```python
from build123d import *

# Parameters (mm, degrees)
SKETCH1_W           = 25.4
SKETCH1_H           = 25.4
BOSS_EXTRUDE1_DEPTH = 107.95
SKETCH2_W           = 22.098
SKETCH2_H           = 22.098
CUT_EXTRUDE1_DEPTH  = 114.769602707
SKETCH3_R           = 3.175
CUT_EXTRUDE2_DEPTH  = 114.769602707


with BuildPart() as part:
    # Sketch1 → Boss-Extrude1 (new body)
    with BuildSketch(Plane(origin=(0, 0, 0), x_dir=(1, 0, 0), z_dir=(0, 1, 0))):
        with Locations((12.7, -12.7)):
            Rectangle(SKETCH1_W, SKETCH1_H)
    extrude(amount=BOSS_EXTRUDE1_DEPTH)

    # Sketch2 → Cut-Extrude1 (cut, through all)
    with BuildSketch(Plane(origin=(0, 107.95, 0), x_dir=(1, 0, 0), z_dir=(0, 1, 0))):
        with Locations((12.7, -12.7)):
            Rectangle(SKETCH2_W, SKETCH2_H)
    extrude(amount=-CUT_EXTRUDE1_DEPTH, mode=Mode.SUBTRACT)

    # Sketch3 → Cut-Extrude2 (cut, through all)
    with BuildSketch(Plane.ZY):
        with Locations((12.7, 12.7)):
            Circle(SKETCH3_R)
    extrude(amount=-CUT_EXTRUDE2_DEPTH, mode=Mode.SUBTRACT)


solid = part.part
```
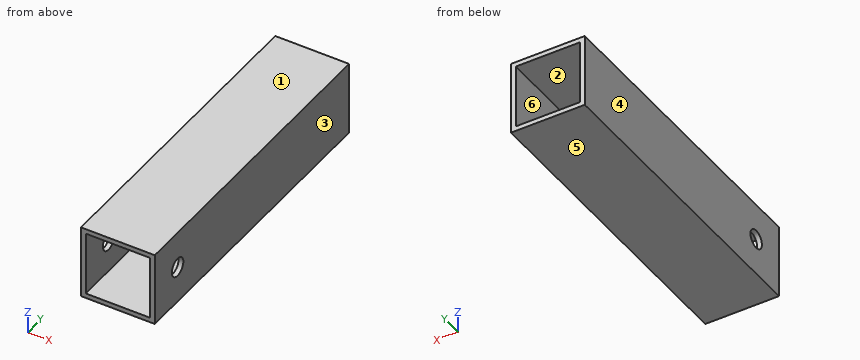
The listing builds one solid part. Answer for the finished solid, in the listing's coordinates (mm). Face numbers are marked on the shaded views. A direction names the side the tool comes from. Coordinates: 2 decimals unless noted, no trailing zeros. Write each loop counter-clockwise with the first axis right and the second up, starting at its lowest first coordinate (ties: lowest second). Pieces come first, ordered by that corner, then holes. Notation, with made-up numbers: (7.5, 81.5) - (62.5, 81.5) arc R8 ccw to (62.5, 92.5) - close; hole circle Ø1 at (-18, 25.25). An arc over 180 degrees is marked (long way). Return JSON: item names as keys, results as strings. Group by question number.
Q1. The part is cut by section C-C on z = 12.7. Write down the section's boundary in (x, y) (3 decimals), and give its area (3 significant figures).
Q2. Find the intervals of material crossed by line 1 along Z through (x, y) = (4.25, 21); line 2 along Y through (x, z) = (0.8, 12.7) (3 decimals), in increasing order. Write a range as [from, to].
Q3. A flat-ended cylindrical pin translates along its axis: pin 1 Ø3 at (x, z) = (21, 3.5) entering from -Y. Find the tip coordinate at first contact, or state that the pin passes through.
Q4. The part is cut by section A-A on z = 22.5. Write down the section's boundary in (x, y).
Q5. Which of the six approach directions +Z, -Z, +X, -X, +Y, -Y give full straight-line access (tool end or side, diameter ignored) to the marked faces 1 and 2?
Q6. For a pull along X with two mould halves and no side action, classify the marked faces 3, 4, 5 and 6 as +X half, -X half, draft (parallel to the pull), parting line (faces both ways), or undercut.
Q7. The part is cut by section D-D on x = 21. Write down the section's boundary in (y, z), and give its area (3 significant figures).
Q8. The part is cut by section B-B on y = 12.7. Write down the section's boundary in (x, z) (3 decimals).
Evaluation:
{
 "1": {"outline": "(0, 0) - (1.651, 0) - (1.651, 9.525) - (0, 9.525) - close; (0, 15.875) - (1.651, 15.875) - (1.651, 107.95) - (0, 107.95) - close; (23.749, 0) - (25.4, 0) - (25.4, 9.525) - (23.749, 9.525) - close; (23.749, 15.875) - (25.4, 15.875) - (25.4, 107.95) - (23.749, 107.95) - close", "area": "335 mm2"},
 "2": {"line 1": "z = [0, 1.65], [23.75, 25.4]", "line 2": "y = [0, 9.525], [15.875, 107.95]"},
 "3": {"pin 1": "passes through"},
 "4": {"outline": "(0, 0) - (1.65, 0) - (1.65, 107.95) - (0, 107.95) - close; (23.75, 0) - (25.4, 0) - (25.4, 107.95) - (23.75, 107.95) - close"},
 "5": {"face 1": "+Z, +X, -X, +Y, -Y", "face 2": "+Y, -Y"},
 "6": {"face 3": "+X half", "face 4": "-X half", "face 5": "draft", "face 6": "undercut"},
 "7": {"outline": "(0, 0) - (107.95, 0) - (107.95, 1.65) - (0, 1.65) - close; (0, 23.75) - (107.95, 23.75) - (107.95, 25.4) - (0, 25.4) - close", "area": "356 mm2"},
 "8": {"outline": "(0, 0) - (25.4, 0) - (25.4, 9.525) - (23.749, 9.525) - (23.749, 1.651) - (1.651, 1.651) - (1.651, 9.525) - (0, 9.525) - close; (0, 15.875) - (1.651, 15.875) - (1.651, 23.749) - (23.749, 23.749) - (23.749, 15.875) - (25.4, 15.875) - (25.4, 25.4) - (0, 25.4) - close"}
}
